Print and shaded views of the part. All mm, measured from the part's lowest x, y and z. Coordinates: 2 decimals unless noted, no trailing zeros. Loops run counter-clockwise (first coordinate to the right, second up) from the corner with the lowest first, then second, coordinate; pieces in that order, holes last. Notation, with made-up numbers: (12, -5) -> (22, -5) arc R16 ccw to (22, 4) -> close; hole circle Ø8 at (82, 4). An arc over 180 degrees is marked (long way). One line per question, with ' | ' between items. Start each with the question number.
1) Cut at C-C (y = 55). List the corners of the cut face in (x, z), plus the area to 3 significant figures.
2) Cut at A-A (x = 47.5). List the corners of the cut face in (y, z).
3) Probe L1, parallel to Z at x = 23, y = 10; L2, parallel to X at y = 15, z = 110.5; L3, parallel to Z at x = 26, y = 46.5. List the from-to ranges inside material, lowest first. Write a range as from..to.
4) Cut at D-D (x = 27). List the corners of the cut face in (y, z), plus the area to 3 significant figures.
5) Drop a flat-ended pin along its axis: pin 1 (20 mm diameter, centred on x = 30.5, y = 20, fed in from +Z). Give the stop position or say it passes through.
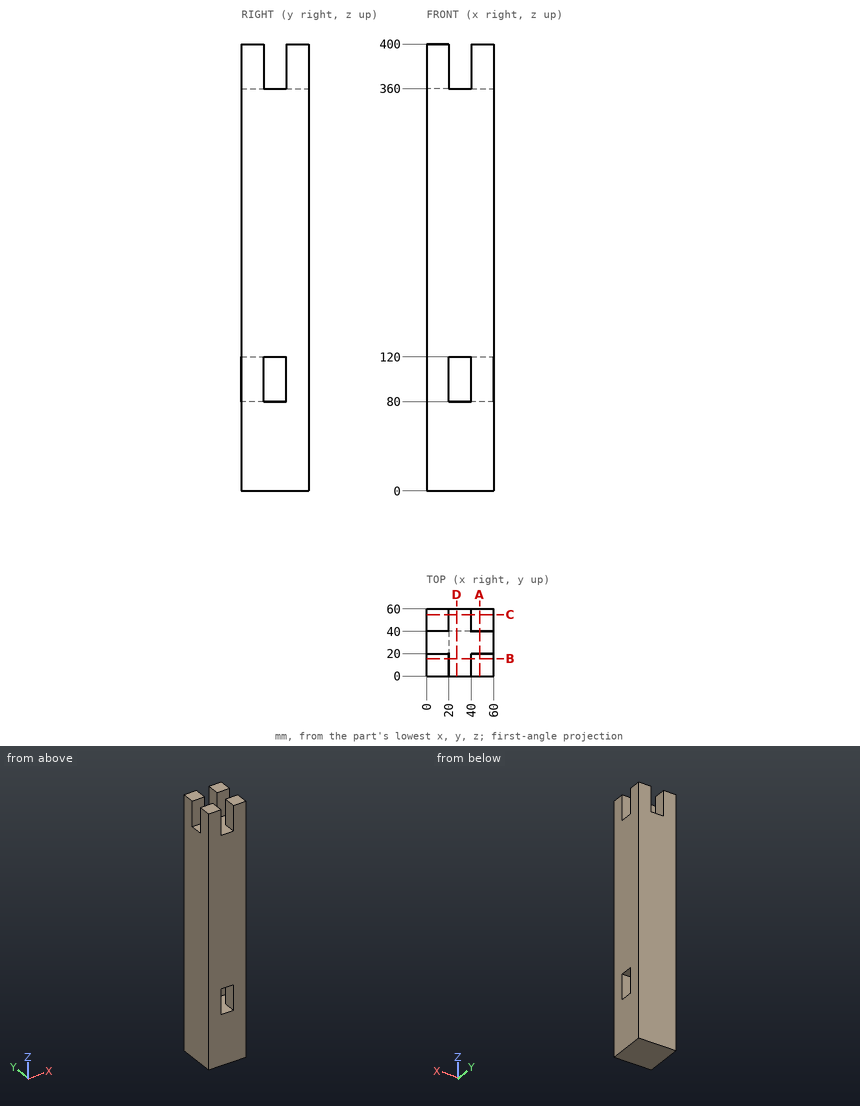
Reported:
1) outline: (0, 0) -> (60, 0) -> (60, 400) -> (40, 400) -> (40, 360) -> (20, 360) -> (20, 400) -> (0, 400) -> close | area: 23,200 mm²
2) outline: (0, 0) -> (60, 0) -> (60, 400) -> (40, 400) -> (40, 360) -> (20, 360) -> (20, 400) -> (0, 400) -> close; hole (20, 80) -> (40, 80) -> (40, 120) -> (20, 120) -> close
3) L1: z = 0..80, 120..360 | L2: x = 0..20, 40..60 | L3: z = 0..360
4) outline: (0, 0) -> (60, 0) -> (60, 360) -> (0, 360) -> (0, 120) -> (40, 120) -> (40, 80) -> (0, 80) -> close | area: 20,000 mm²
5) pin 1: stops at z = 400
